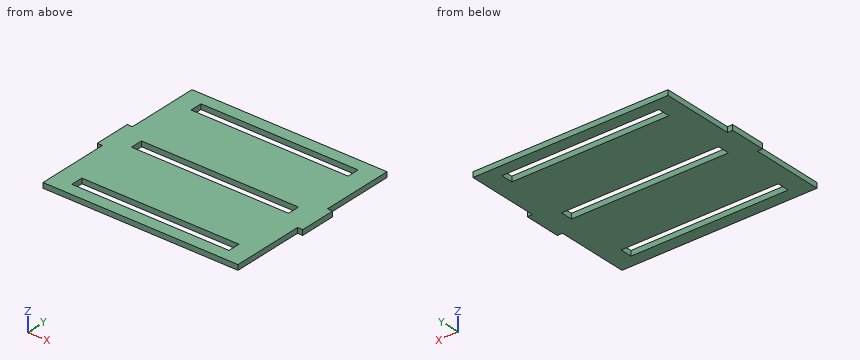
```python
from build123d import *

# Parameters (mm, degrees)
SKETCH1_W           = 130
SKETCH1_H           = 10
BOSS_EXTRUDE1_DEPTH = 4.3


with BuildPart() as part:
    # Sketch1 → Boss-Extrude1 (new body)
    with BuildSketch(Plane.XY):
        Polygon((80.7, 15.1), (80.7, 75), (-80.7, 75), (-80.7, 15.1), (-85, 15.1), (-85, -15.1), (-80.7, -15.1), (-80.7, -75), (80.7, -75), (80.7, -15.1), (85, -15.1), (85, 15.1), align=None)
        with Locations((0, 60)):
            Rectangle(SKETCH1_W, SKETCH1_H, mode=Mode.SUBTRACT)
        Rectangle(SKETCH1_W, SKETCH1_H, mode=Mode.SUBTRACT)
        with Locations((0, -60)):
            Rectangle(SKETCH1_W, SKETCH1_H, mode=Mode.SUBTRACT)
    extrude(amount=BOSS_EXTRUDE1_DEPTH)


solid = part.part
```
Check sheet for the modelled part. Datum: model origin and axes. Units: mm. Round coordinates to 2 decimals unless told otherwise and drop trailing zeros. Write each loop counter-clockwise with the first axis right and the second up, starting at its lowest first coordinate (ties: lowest second). Pieces come first, ordered by that corner, then holes. Notation, with made-up numbers: (86, 19.5) -> (93, 19.5) arc R20 ccw to (93, 25.5) -> close; hole circle Ø8 at (88, 42.5). An arc over 180 degrees is marked (long way). One line per question, with ' | ' between items. Start each with the question number.
1. Sectioned sample at B-B, the plane z = 0.85. Record the cut outline in (x, y), then the cut area to 3 significant figures.
2. Sectioned sample at A-A, the plane x = -26. Record the cut outline in (y, z).
3. Scan lines: line 1 along Y through (x, z) = (-25, 1.75); line 2 along X through (y, z) = (-62, 3.45); line 3 along X through (y, z) = (-3, 1.75). Record each from-to range of solid material in increasing order. Write a range as from..to.
4. Sectioned sample at C-C, the plane y = 18.5. Record the cut outline in (x, z).
5. Depth check by flat-ended pin: pin 1 (1.3 mm diameter, centred on x = 82.5, z = 3, fed in from -Y); pin 2 (1.3 mm diameter, centred on y = 46, z = 2, fed in from +X); pin 3 (2 mm diameter, centred on y = -62, z = 2.5, fed in from -X); pin 4 (10 mm diameter, centred on x = 59, y = 4.5, fed in from +Z). Enter the tip coordinate at first touch or a pass-through.
Taken from the geometry:
1) outline: (-85, -15.1) -> (-80.7, -15.1) -> (-80.7, -75) -> (80.7, -75) -> (80.7, -15.1) -> (85, -15.1) -> (85, 15.1) -> (80.7, 15.1) -> (80.7, 75) -> (-80.7, 75) -> (-80.7, 15.1) -> (-85, 15.1) -> close; hole (-65, -65) -> (65, -65) -> (65, -55) -> (-65, -55) -> close; hole (-65, -5) -> (65, -5) -> (65, 5) -> (-65, 5) -> close; hole (-65, 55) -> (65, 55) -> (65, 65) -> (-65, 65) -> close | area: 20,600 mm^2
2) outline: (-75, 0) -> (-65, 0) -> (-65, 4.3) -> (-75, 4.3) -> close; (-55, 0) -> (-5, 0) -> (-5, 4.3) -> (-55, 4.3) -> close; (5, 0) -> (55, 0) -> (55, 4.3) -> (5, 4.3) -> close; (65, 0) -> (75, 0) -> (75, 4.3) -> (65, 4.3) -> close
3) line 1: y = -75..-65, -55..-5, 5..55, 65..75 | line 2: x = -80.7..-65, 65..80.7 | line 3: x = -85..-65, 65..85
4) outline: (-80.7, 0) -> (80.7, 0) -> (80.7, 4.3) -> (-80.7, 4.3) -> close
5) pin 1: stops at y = -15.1 | pin 2: stops at x = 80.7 | pin 3: stops at x = -80.7 | pin 4: stops at z = 4.3
